Here's how the part is built. I have some questions about the finished solid (model axes, mm). A direction names the side the tool comes from. Coordinates: 2 decimals unless noted, no trailing zeros. Write each loop counter-clockwise with the first axis right and the second up, starting at its lowest first coordinate (ties: lowest second). Pieces come first, ordered by that corner, then holes. Notation, with made-up numbers: (2.5, -33.75) -> (51.5, -33.75) arc R23 cw to (51.5, -1.75) -> close; hole circle Ø9 at (-9, 79). An arc over 180 degrees is marked (long way). Use CSV: the item, a comma, the result in double quotes. Start each with the question number.
```python
from build123d import *

# Parameters (mm, degrees)
BOSS_EXTRUDE1_DEPTH      = 25.4
BOSS_EXTRUDE2_DEPTH      = 25.4
BOSS_EXTRUDE3_DEPTH      = 152.4
BOSS_EXTRUDE4_DEPTH      = 12.7
BOSS_EXTRUDE4_DEPTH_BACK = 12.7
SKETCH5_R                = 38.1
SKETCH5_R_2              = 19.05
CUT_EXTRUDE1_DEPTH       = 981.124094184
CUT_EXTRUDE2_DEPTH       = 25.4
SCALE1_SCALE             = 2.84


with BuildPart() as part:
    # Sketch1 → Boss-Extrude1 (new body)
    with BuildSketch(Plane.XY):
        Polygon((-914.4, 304.8), (-812.8, 304.8), (0, 254), (0, 0), (-177.8, 0), (-812.8, 203.2), (-914.4, 203.2), align=None)
    extrude(amount=-BOSS_EXTRUDE1_DEPTH)



with BuildPart() as body_2:
    # Sketch2 → Boss-Extrude2 (new body)
    with BuildSketch(Plane.XY.offset(127)):
        Polygon((-812.8, 203.2), (-177.8, 0), (0, 0), (0, 254), (-812.8, 304.8), (-914.4, 304.8), (-914.4, 203.2), align=None)
    extrude(amount=BOSS_EXTRUDE2_DEPTH)


with BuildPart() as part_1:
    add(part.part)

    add(body_2.part)  # Boss-Extrude3 merges body 2
    # Sketch3 → Boss-Extrude3 (add)
    with BuildSketch(Plane.XY.offset(152.4)):
        Polygon((-914.4, 279.4), (-914.4, 304.8), (-812.8, 304.8), (0, 254), (0, 228.550438977), (-25.4, 230.137938977), (-813.592976364, 279.4), align=None)
    extrude(amount=-BOSS_EXTRUDE3_DEPTH)

    # Sketch6 → Boss-Extrude4 (add, two sides: drawn at the far end of the back side and taken through both)
    with BuildSketch(Plane.XY.offset(63.5).offset(-BOSS_EXTRUDE4_DEPTH_BACK)):
        Polygon((-812.8, 203.2), (-177.8, 0), (0, 0), (0, 254), (-812.8, 304.8), (-914.4, 304.8), (-914.4, 203.2), align=None)
    extrude(amount=BOSS_EXTRUDE4_DEPTH + BOSS_EXTRUDE4_DEPTH_BACK)

    # Sketch5 → Cut-Extrude1 (cut, through all)
    with BuildSketch(Plane.XY.offset(152.4)):
        with Locations((-63.5, 168.969627955)):
            Circle(SKETCH5_R)
        with Locations((-171.45, 44.45)):
            Circle(SKETCH5_R_2)
    extrude(amount=-CUT_EXTRUDE1_DEPTH, mode=Mode.SUBTRACT)

    # Sketch7 → Cut-Extrude2 (cut)
    with BuildSketch(Plane.XY.offset(76.2)):
        Polygon((-475.45625, 95.25), (0, 95.25), (0, 0), (-177.8, 0), align=None)
    extrude(amount=-CUT_EXTRUDE2_DEPTH, mode=Mode.SUBTRACT)


with BuildPart() as part_2:
    # Scale1: scaled about (-409.969923115, 196.838960964, 63.5)
    add(part_1.part.scale(SCALE1_SCALE).moved(Location((754.344658532, -362.183688174, -116.84))))


solid = part_2.part
```
Item 1: I want a section at D-D on x = -1296. Please give me the cut outline in (y, z), then the cut area to 3 significant figures.
Item 2: I'm going to push flat-ended pins straight in: pin 1 (6 mm diameter, centred on x = -1129.5, z = 264.5, fed in from -Y); pin 2 (12 mm diameter, centred on x = -1293.5, z = 27.5, fed in from +Y); pin 3 (21.5 mm diameter, centred on x = -1710.5, z = 80, fed in from -Y). Where does each tip first touch, or does it pass through?
Item 3: I want a section at A-A on y = 256. Please give me the cut outline in (x, z), then the cut area to 3 significant figures.
Item 4: I want a section at C-C on z = -157. Please give me the cut outline in (x, y), then the cut area to 3 significant figures.
Item 5: Thinking about a two-plate mould opening in Z: for faces 1 (the flat face through (-639.68, -77.68, -152.4)), 2 (the flat face through (-274, 173, 315.976)), 3 (the flat face through (-417.132, 360.117, 172.714)), which applies, +Z half, -Z half, draft (parallel to the pull), parting line (faces both ways), or undercut?
Item 6: Which directions (+Z, -Z, +X, -X, +Y, -Y) give clear straight access to the entire face, cutting with the end or side of a thin tool? Please do faces 4 (the flat face through (70, -91.674, 64)), 5 (the flat face through (-274, 128, 243.84)), 6 (the flat face through (-1700, 214.904, 279)), 7 (the cylindrical face through (465.905, 122.448, 64.005)).
Item 7: If I drill on line 1 along Z through (x, y) = (-637, -22.5); line 2 along Y through (x, z) = (-1679, 89); line 3 along Y through (x, z) = (-1705, -111.5), over which ranges is the centre line in solid material (lowest first)?
Item 8: I want a section at B-B on z = -25. Please give me the cut outline in (x, y).
Geometry says:
1,outline,"(132.34, -188.98) -> (487.32, -188.98) -> (487.32, 315.98) -> (132.34, 315.98) -> (132.34, 243.84) -> (415.05, 243.84) -> (415.05, 99.57) -> (132.34, 99.57) -> (132.34, 27.43) -> (415.05, 27.43) -> (415.05, -116.84) -> (132.34, -116.84) -> close"
1,area,"97,700 mm2"
2,pin 1,"y = 78.1"
2,pin 2,"y = 487.54"
2,pin 3,"y = 214.9"
3,outline,"(-1842.55, -188.98) -> (754.34, -188.98) -> (754.34, -116.84) -> (-1842.55, -116.84) -> close; (-1842.55, 27.43) -> (754.34, 27.43) -> (754.34, 99.57) -> (-1842.55, 99.57) -> close; (-1842.55, 243.84) -> (754.34, 243.84) -> (754.34, 315.98) -> (-1842.55, 315.98) -> close"
3,area,"562,000 mm2"
4,outline,"(-1842.55, 214.9) -> (-1554.01, 214.9) -> (249.39, -362.18) -> (754.34, -362.18) -> (754.34, 359.18) -> (-1554.01, 503.45) -> (-1842.55, 503.45) -> close; hole circle Ø108.2 at (267.43, -235.95); hole circle Ø216.41 at (574, 117.69)"
4,area,"1,350,000 mm2"
5,face 1,"draft"
5,face 2,"+Z half"
5,face 3,"undercut"
6,face 4,"+X, -X, -Y"
6,face 5,"-X, -Y"
6,face 6,"+Z, -Z, -X, -Y"
6,face 7,"+Z, -Z"
7,line 1,"-188.98 to -116.84, 27.43 to 99.57, 243.84 to 315.98"
7,line 2,"214.9 to 503.45"
7,line 3,"431.31 to 503.45"
8,outline,"(-1842.55, 431.31) -> (-1556.26, 431.31) -> (754.34, 286.9) -> (754.34, 359.18) -> (-1554.01, 503.45) -> (-1842.55, 503.45) -> close"
